```python
from build123d import *

# Parameters (mm, degrees)
BOSS_EXTRUDE1_DEPTH             = 3
M3_CLEARANCE_HOLE1_D            = 3.4
BOSS_EXTRUDE3_DEPTH             = 13
BOSS_EXTRUDE3_DEPTH_BACK        = 13
BOSS_EXTRUDE4_REACH             = 52.335
BOSS_EXTRUDE4_DIRECTION_2_REACH = 52.335
CUT_EXTRUDE1_REACH              = 52.395
SKETCH7_R                       = 3.25


with BuildPart() as part:
    # Sketch1 → Boss-Extrude1 (new body)
    with BuildSketch(Plane.XY):
        with BuildLine():
            Line((-40.923076923, -5.115384615), (-3.076923077, -5.115384615))
            ThreePointArc((-3.076923077, -5.115384615), (-0.839748528, -3.273500981), (0, -0.5))
            Line((0, -0.5), (0, 10.5))
            Line((0, 10.5), (-2, 12.5))
            Line((-2, 12.5), (-42, 12.5))
            Line((-42, 12.5), (-44, 10.5))
            Line((-44, 10.5), (-44, -0.5))
            ThreePointArc((-44, -0.5), (-43.160251472, -3.273500981), (-40.923076923, -5.115384615))
        make_face()
    extrude(amount=BOSS_EXTRUDE1_DEPTH)

    # M3 Clearance Hole1 (through all)
    with Locations(Plane.XY.offset(3)):
        with Locations((-37, 7.5), (-37, -1.5), (-7, 7.5), (-7, -1.5)):
            Hole(M3_CLEARANCE_HOLE1_D / 2)

    # Sketch5 → Boss-Extrude3 (add, two sides: drawn at the far end of the back side and taken through both)
    with BuildSketch(Plane(origin=(-22, 0, 0), x_dir=(0, 0, -1), z_dir=(1, 0, 0)).offset(-BOSS_EXTRUDE3_DEPTH_BACK)):
        Polygon((-18, 12.5), (-21.106067583, -5.115384615), (-3, -5.115384615), (-3, 12.5), align=None)
    extrude(amount=BOSS_EXTRUDE3_DEPTH + BOSS_EXTRUDE3_DEPTH_BACK)

    # Boss-Extrude4: up to this plane
    boss_extrude4_end = Plane(origin=(-40.923076923, -5.115384615, 3), z_dir=(0, 1, 0))
    # Sketch6 → Boss-Extrude4 (add, up to the surface)
    with BuildSketch(Plane(origin=(0, 0.237205282, -0.041825691), x_dir=(1, 0, 0), z_dir=(0, 0.9848077530122074, -0.17364817766693444)), mode=Mode.PRIVATE) as boss_extrude4_sk1:
        Polygon((-35, -19.897141775), (-35, -21.397141775), (-33.5, -22.897141775), (-27.15, -22.897141775), (-30.15, -19.897141775), align=None)
    boss_extrude4_tool1 = split(extrude(boss_extrude4_sk1.sketch, amount=-BOSS_EXTRUDE4_REACH, mode=Mode.PRIVATE), bisect_by=boss_extrude4_end, keep=Keep.BOTH, mode=Mode.PRIVATE)
    add(boss_extrude4_tool1.solids().sort_by_distance((-31.594351, 3.963678, 21.092053))[0])
    # Sketch6 → Boss-Extrude4 (add, up to the surface)
    with BuildSketch(Plane(origin=(0, 0.237205282, -0.041825691), x_dir=(1, 0, 0), z_dir=(0, 0.9848077530122074, -0.17364817766693444)), mode=Mode.PRIVATE) as boss_extrude4_sk2:
        Polygon((-13.85, -19.897141775), (-16.85, -22.897141775), (-10.5, -22.897141775), (-9, -21.397141775), (-9, -19.897141775), align=None)
    boss_extrude4_tool2 = split(extrude(boss_extrude4_sk2.sketch, amount=-BOSS_EXTRUDE4_REACH, mode=Mode.PRIVATE), bisect_by=boss_extrude4_end, keep=Keep.BOTH, mode=Mode.PRIVATE)
    add(boss_extrude4_tool2.solids().sort_by_distance((-12.405649, 3.963678, 21.092053))[0])

    # Boss-Extrude4 direction 2: up to this plane
    boss_extrude4_direction_2_end = Plane(origin=(-2, 12.5, 3), z_dir=(0, -1, 0))
    # Sketch6 → Boss-Extrude4 direction 2 (add, up to the surface)
    with BuildSketch(Plane(origin=(0, 0.237205282, -0.041825691), x_dir=(1, 0, 0), z_dir=(0, 0.9848077530122074, -0.17364817766693444)), mode=Mode.PRIVATE) as boss_extrude4_direction_2_sk1:
        Polygon((-35, -19.897141775), (-35, -21.397141775), (-33.5, -22.897141775), (-27.15, -22.897141775), (-30.15, -19.897141775), align=None)
    boss_extrude4_direction_2_tool1 = split(extrude(boss_extrude4_direction_2_sk1.sketch, amount=BOSS_EXTRUDE4_DIRECTION_2_REACH, mode=Mode.PRIVATE), bisect_by=boss_extrude4_direction_2_end, keep=Keep.BOTH, mode=Mode.PRIVATE)
    add(boss_extrude4_direction_2_tool1.solids().sort_by_distance((-31.594351, 3.963678, 21.092053))[0])
    # Sketch6 → Boss-Extrude4 direction 2 (add, up to the surface)
    with BuildSketch(Plane(origin=(0, 0.237205282, -0.041825691), x_dir=(1, 0, 0), z_dir=(0, 0.9848077530122074, -0.17364817766693444)), mode=Mode.PRIVATE) as boss_extrude4_direction_2_sk2:
        Polygon((-13.85, -19.897141775), (-16.85, -22.897141775), (-10.5, -22.897141775), (-9, -21.397141775), (-9, -19.897141775), align=None)
    boss_extrude4_direction_2_tool2 = split(extrude(boss_extrude4_direction_2_sk2.sketch, amount=BOSS_EXTRUDE4_DIRECTION_2_REACH, mode=Mode.PRIVATE), bisect_by=boss_extrude4_direction_2_end, keep=Keep.BOTH, mode=Mode.PRIVATE)
    add(boss_extrude4_direction_2_tool2.solids().sort_by_distance((-12.405649, 3.963678, 21.092053))[0])

    # Sketch7 → Cut-Extrude1 (cut, up to next)
    with BuildSketch(Plane.XY.offset(3), mode=Mode.PRIVATE) as cut_extrude1_sk1:
        with Locations((-37, 7.5)):
            Circle(SKETCH7_R)
    cut_extrude1_tool1 = extrude(cut_extrude1_sk1.sketch, amount=CUT_EXTRUDE1_REACH, mode=Mode.PRIVATE) & part.part
    # Sketch7 → Cut-Extrude1 (cut, up to next)
    with BuildSketch(Plane.XY.offset(3), mode=Mode.PRIVATE) as cut_extrude1_sk2:
        with Locations((-37, -1.5)):
            Circle(SKETCH7_R)
    cut_extrude1_tool2 = extrude(cut_extrude1_sk2.sketch, amount=CUT_EXTRUDE1_REACH, mode=Mode.PRIVATE) & part.part
    # Sketch7 → Cut-Extrude1 (cut, up to next)
    with BuildSketch(Plane.XY.offset(3), mode=Mode.PRIVATE) as cut_extrude1_sk3:
        with Locations((-7, -1.5)):
            Circle(SKETCH7_R)
    cut_extrude1_tool3 = extrude(cut_extrude1_sk3.sketch, amount=CUT_EXTRUDE1_REACH, mode=Mode.PRIVATE) & part.part
    # Sketch7 → Cut-Extrude1 (cut, up to next)
    with BuildSketch(Plane.XY.offset(3), mode=Mode.PRIVATE) as cut_extrude1_sk4:
        with Locations((-7, 7.5)):
            Circle(SKETCH7_R)
    cut_extrude1_tool4 = extrude(cut_extrude1_sk4.sketch, amount=CUT_EXTRUDE1_REACH, mode=Mode.PRIVATE) & part.part
    add(cut_extrude1_tool1.solids().sort_by_distance((-37, 7.5, 3))[0], mode=Mode.SUBTRACT)
    add(cut_extrude1_tool2.solids().sort_by_distance((-37, -1.5, 3))[0], mode=Mode.SUBTRACT)
    add(cut_extrude1_tool3.solids().sort_by_distance((-7, -1.5, 3))[0], mode=Mode.SUBTRACT)
    add(cut_extrude1_tool4.solids().sort_by_distance((-7, 7.5, 3))[0], mode=Mode.SUBTRACT)


solid = part.part
```
Check sheet for the modelled part. Datum: model origin and axes. Units: mm. A direction names the side the tool comes from. Round coordinates to 2 decimals unless told otherwise and drop trailing zeros. Loops run counter-clockwise (first coordinate to the right, second up) from the corner with the lowest first, then second, coordinate; pieces in that order, holes last. Notation, with made-up numbers: (64.5, 13.25) - (104.5, 13.25) arc R28 ccw to (104.5, 51.25) - close; hole circle Ø4 at (17.5, 32). An arc over 180 degrees is marked (long way). Answer as a JSON object with one key per item and string values. Group by question number.
Q1. Mould release check, pull along Y, two halves, no side actions. Record for faces 5 (the face through (-30.37, 3.57, 22.62)), 6 (the face through (-33.75, -1.54, 13.03)), 7 (the face through (0, 5, 1)): released by +Y, released by -Y, zero draft, split by the parting line, or undercut.
Q2. Sectioned sample at A-A, the plane z = 2.5. Enter the section's corners in (x, y).
Q3. Set-up check for faces 1 (the face through (-10.25, 7.54, 12.32)), 2 (the face through (-33.75, 7.46, 12.25)), 3 (the face through (-34.094, 3.594, 22.014)), 4 (the face through (-9, 3, 12)): record each of +Z, -Z, +X, -X, +Y, -Y from which the full face is reachable in a straight line by a thin tool's end or side.
Q4. Sectioned sample at B-B, the plane x = -37. Enter the section's corners in (y, z), plus the area to 3 significant figures.
Q5. Sectioned sample at C-C, the plane y = -2. Enter the section's corners in (x, z), plus the area to 3 significant figures.
Q6. Sectioned sample at D-D, the plane x = -11. Enter the section's corners in (y, z), plus the area to 3 significant figures.
Q7. Gauge pin test, flat ends, axial feed: P1, Ø0.5, axis at y = -4.5, z = 13.5, coming from the -X side; P2, Ø4, axis at x = -15, y = 7.5, coming from the +Z side; P3, Ø5, axis at x = -4.5, y = 1, coming from the +Z side; P4, Ø1.5, axis at x = -7, z = 8, coming from the +Y side. Record the tip position at first contact, or that the pin passes through.
Q8. Scan lines: line 1 along Y through (x, z) = (-37, 2.3); line 2 along X through (y, z) = (1.5, 14.75); line 3 along X through (y, z) = (-3.75, 21). Record each from-to range of solid material in increasing order. Write a range as [from, to].
Solution:
{
 "1": {"face 5": "released by +Y", "face 6": "undercut", "face 7": "zero draft"},
 "2": {"outline": "(-44, -0.5) arc R5 ccw to (-40.92, -5.12) - (-3.08, -5.12) arc R5 ccw to (0, -0.5) - (0, 10.5) - (-2, 12.5) - (-42, 12.5) - (-44, 10.5) - close; hole circle Ø3.4 at (-37, -1.5); hole circle Ø3.4 at (-37, 7.5); hole circle Ø3.4 at (-7, -1.5); hole circle Ø3.4 at (-7, 7.5)"},
 "3": {"face 1": "+Z, +X", "face 2": "+Z, -X", "face 3": "+Z, -X, +Y", "face 4": "+Z, +X, +Y, -Y"},
 "4": {"outline": "(-5.12, 0) - (-3.2, 0) - (-3.2, 3) - (-5.12, 3) - close; (0.2, 0) - (5.8, 0) - (5.8, 3) - (0.2, 3) - close; (9.2, 0) - (12.5, 0) - (12.5, 3) - (9.2, 3) - close", "area": "32.4 mm²"},
 "5": {"outline": "(-43.77, 0) - (-38.62, 0) - (-38.62, 3) - (-43.77, 3) - close; (-35.38, 0) - (-8.62, 0) - (-8.62, 3) - (-10.21, 3) - (-10.21, 23.31) - (-10.5, 23.6) - (-16.85, 23.6) - (-13.85, 20.56) - (-30.15, 20.56) - (-27.15, 23.6) - (-33.5, 23.6) - (-33.79, 23.31) - (-33.79, 3) - (-35.38, 3) - close; (-5.38, 0) - (-0.23, 0) - (-0.23, 3) - (-5.38, 3) - close", "area": "556 mm²"},
 "6": {"outline": "(-5.12, 0) - (12.5, 0) - (12.5, 21.05) - (-5.12, 24.15) - close", "area": "398 mm²"},
 "7": {"P1": "stops at x = -35", "P2": "stops at z = 22.28", "P3": "stops at z = 3", "P4": "passes through"},
 "8": {"line 1": "y = [-5.12, -3.2], [0.2, 5.8], [9.2, 12.5]", "line 2": "x = [-35, -9]", "line 3": "x = [-34.65, -30.02], [-13.98, -9.35]"}
}
